Design review of the part built by this model. Coordinates are the model's own, in mm. A direction names the side the tool comes from. Coordinates: 2 decimals unless noted, no trailing zeros. Loops run counter-clockwise (first coordinate to the right, second up) from the corner with the lowest first, then second, coordinate; pieces in that order, holes last. Notation, with made-up numbers: (53.5, 29.5) - (91.5, 29.5) arc R29 cw to (91.5, 58.5) - close; hole circle Ø7 at (-34, -39.5). An arc over 180 degrees is marked (long way). Answer in a Markdown table with one row per item. Add a question column.
(1) To check wall thickness, follow L1, parallel to Y at x = 0, z = -22; L2, parallel to X at y = 73, z = -17.5. State the ranges of each line that lie inside material, in increasing order. Write a range as [from, to].
(2) For faces 1 (the face through (3.86, -9.39, -5.04)), 2 (the face through (-25.4, 44, 0)), 3 (the face through (-5, 49, -19.05)), list the 3-axis set-ups (+Z, -Z, +X, -X, +Y, -Y) from which the entire face can be reached by the end or side of a thin tool; tool diameter is ignored.
(3) The part is to be moulded in two halves that separate along Y. For faces 4 (the face through (22, 88.9, 0)), 5 (the face through (19.05, 49, 0)), 6 (the face through (-3.51, 55.146, 22.269)), say which applies: released by +Y, released by -Y, zero draft, split by the parting line, or undercut.
(4) We need section D-D, the plane z = -10.5. Write out the cut boundary in (x, y), plus the area to 3 significant figures.
(5) Clearance check with flat-ended pins moving along their axes: pin 1 (5.5 mm diameter, centred on x = 0, y = 70.98, fed in from +Z); pin 2 (6 mm diameter, centred on x = -6, z = 9, fed in from -Y); pin 3 (15 mm diameter, centred on x = 0, y = 51.93, fed in from -Z); pin 4 (19 mm diameter, centred on x = 2, z = 4.5, fed in from +Y). State where each tip first meets the part, or that it passes through.
(6) We need section C-C, the plane y = 12.5. Write out the cut boundary in (x, z).
(7) We need section B-B, the plane x = 0. Give the number of separate pieces and of enclosed holes in the cut face, plus the area to 3 significant figures.
(8) We need section A-A, the plane y = 55. Write out the cut boundary in (x, z), plus the area to 3 significant figures.
from build123d import *

# Parameters (mm, degrees)
SKETCH1_W           = 50.8
SKETCH1_H           = 50.8
BOSS_EXTRUDE1_DEPTH = 88.9
SKETCH2_W           = 38.1
SKETCH2_H           = 38.1
CUT_EXTRUDE1_DEPTH  = 96.882897328
SKETCH3_W           = 38.1
SKETCH3_H           = 38.1
BOSS_EXTRUDE2_DEPTH = 7.62
SKETCH4_R           = 6.35
BOSS_EXTRUDE3_DEPTH = 19.05
SKETCH6_R           = 4.7625
CUT_EXTRUDE2_DEPTH  = 106.494123059


with BuildPart() as part:
    # Sketch1 → Boss-Extrude1 (new body)
    with BuildSketch(Plane(origin=(0, 0, 0), x_dir=(1, 0, 0), z_dir=(0, 1, 0))):
        Rectangle(SKETCH1_W, SKETCH1_H)
    extrude(amount=BOSS_EXTRUDE1_DEPTH)

    # Sketch2 → Cut-Extrude1 (cut, through all)
    with BuildSketch(Plane(origin=(0, 88.9, 0), x_dir=(1, 0, 0), z_dir=(0, 1, 0))):
        Rectangle(SKETCH2_W, SKETCH2_H)
    extrude(amount=-CUT_EXTRUDE1_DEPTH, mode=Mode.SUBTRACT)

    # Sketch3 → Boss-Extrude2 (add)
    with BuildSketch(Plane(origin=(0, 0, 0), x_dir=(-1, 0, 0), z_dir=(0, -1, 0))):
        Rectangle(SKETCH3_W, SKETCH3_H)
    extrude(amount=-BOSS_EXTRUDE2_DEPTH)

    # Sketch4 → Boss-Extrude3 (add)
    with BuildSketch(Plane(origin=(0, 0, 0), x_dir=(-1, 0, 0), z_dir=(0, -1, 0))):
        with Locations(Location((0, 0, 0), (0, 0, 270))):
            Circle(SKETCH4_R)
    extrude(amount=BOSS_EXTRUDE3_DEPTH)

    # Sketch6 → Cut-Extrude2 (cut, through all)
    with BuildSketch(Plane.XY.offset(25.4)):
        with Locations((0, 70.977272932)):
            Circle(SKETCH6_R)
        with Locations((0, 51.927272932)):
            Circle(SKETCH6_R)
        with Locations((0, 32.877272932)):
            Circle(SKETCH6_R)
    extrude(amount=-CUT_EXTRUDE2_DEPTH, mode=Mode.SUBTRACT)


solid = part.part
Responses:
| question | item | result |
|---|---|---|
| 1 | L1 | y = [0, 28.11], [37.64, 47.16], [56.69, 66.21], [75.74, 88.9] |
| 1 | L2 | x = [-25.4, -19.05], [19.05, 25.4] |
| 2 | face 1 | -Y |
| 2 | face 2 | +Z, -Z, -X, +Y, -Y |
| 2 | face 3 | +Y |
| 3 | face 4 | released by +Y |
| 3 | face 5 | zero draft |
| 3 | face 6 | undercut |
| 4 | outline | (-25.4, 0) - (25.4, 0) - (25.4, 88.9) - (19.05, 88.9) - (19.05, 7.62) - (-19.05, 7.62) - (-19.05, 88.9) - (-25.4, 88.9) - close |
| 4 | area | 1,420 mm2 |
| 5 | pin 1 | passes through |
| 5 | pin 2 | stops at y = 0 |
| 5 | pin 3 | stops at z = -25.4 |
| 5 | pin 4 | stops at y = 7.62 |
| 6 | outline | (-25.4, -25.4) - (25.4, -25.4) - (25.4, 25.4) - (-25.4, 25.4) - close; hole (-19.05, -19.05) - (19.05, -19.05) - (19.05, 19.05) - (-19.05, 19.05) - close |
| 7 | separate pieces | 7 |
| 7 | enclosed holes | 0 |
| 7 | area | 1,300 mm2 |
| 8 | outline | (-25.4, -25.4) - (-3.64, -25.4) - (-3.64, -19.05) - (-19.05, -19.05) - (-19.05, 19.05) - (-3.64, 19.05) - (-3.64, 25.4) - (-25.4, 25.4) - close; (3.64, -25.4) - (25.4, -25.4) - (25.4, 25.4) - (3.64, 25.4) - (3.64, 19.05) - (19.05, 19.05) - (19.05, -19.05) - (3.64, -19.05) - close |
| 8 | area | 1,040 mm2 |
